```python
from build123d import *

# Parameters (mm, degrees)
SM_BASE_FLANGE_1_DEPTH            = 3
SM_EDGE_FLANGE_1_STRIP_W          = 13.4732
SM_EDGE_FLANGE_1_STRIP_H          = 3
SM_EDGE_FLANGE_1_STRIP_CUT_DEPTH  = 65.533094289
SM_EDGE_FLANGE_1_RELIEF_W         = 14.9732
SM_EDGE_FLANGE_1_RELIEF_H         = 1.5
SM_EDGE_FLANGE_1_RELIEF_CUT_DEPTH = 3
SM_EDGE_FLANGE_1_DEPTH            = 65.533094289
CHAMFER_1_SIZE                    = 5
CUT_EXTRUDE_1_DEPTH               = 10


# Sheet-metal steps are written as plain solids
with BuildPart() as part:
    # Sketch 1 → 基体-法兰1 (new body)
    with BuildSketch(Plane.XY):
        Polygon((75, -35), (75, -85.533094289), (95, -85.533094289), (95, 0), (0, 0), (0, -35), align=None)
    extrude(amount=-SM_BASE_FLANGE_1_DEPTH)

    # 边线-法兰1 strip (across the edge) → 边线-法兰1 strip cut (cut)
    with BuildSketch(Plane(origin=(95, -85.533094289, 0), x_dir=(-1, 0, 0), z_dir=(0, 1, 0))):
        with Locations((-3, -1.5)):
            Rectangle(SM_EDGE_FLANGE_1_STRIP_W, SM_EDGE_FLANGE_1_STRIP_H)
    extrude(amount=SM_EDGE_FLANGE_1_STRIP_CUT_DEPTH, mode=Mode.SUBTRACT)

    # 边线-法兰1 relief (on the sheet) → 边线-法兰1 relief cut (cut)
    with BuildSketch(Plane(origin=(91.2634, -85.533094289, 0), x_dir=(-1, 0, 0), z_dir=(0, 0, 1))):
        with Locations((-5.9866, -66.283094289)):
            Rectangle(SM_EDGE_FLANGE_1_RELIEF_W, SM_EDGE_FLANGE_1_RELIEF_H)
    extrude(amount=-SM_EDGE_FLANGE_1_RELIEF_CUT_DEPTH, mode=Mode.SUBTRACT)

    # 边线-法兰1 section (across the edge) → 边线-法兰1 (add)
    with BuildSketch(Plane(origin=(95, -85.533094289, 0), x_dir=(-1, 0, 0), z_dir=(0, 1, 0))):
        with BuildLine():
            Line((0, 0.7366), (0, 27))
            Line((0, 27), (3, 27))
            Line((3, 27), (3, 0.7366))
            ThreePointArc((3, 0.7366), (3.215745145, 0.215745145), (3.7366, 0))
            Line((3.7366, 0), (3.7366, -3))
            ThreePointArc((3.7366, -3), (1.094424801, -1.905575199), (0, 0.7366))
        make_face()
    extrude(amount=SM_EDGE_FLANGE_1_DEPTH)

    # 倒角1
    chamfer_1_edges = [part.edges().sort_by_distance(p)[0] for p in [
        (0, 0, -1.5),
        (95, 0, -1.5),
        (75, -85.533094289, -1.5),
        (0, -35, -1.5),
        (93.5, -85.533094289, 27),
        (93.5, -20, 27),
    ]]
    chamfer(chamfer_1_edges, length=CHAMFER_1_SIZE)

    # 草图10 → 切除-拉伸1 (cut)
    with BuildSketch(Plane.XY):
        with BuildLine():
            Line((11, -14), (19, -14))
            ThreePointArc((19, -14), (22.5, -17.5), (19, -21))
            Line((19, -21), (11, -21))
            ThreePointArc((11, -21), (7.5, -17.5), (11, -14))
        make_face()
        with BuildLine():
            Line((51, -14), (59, -14))
            ThreePointArc((59, -14), (62.5, -17.5), (59, -21))
            Line((59, -21), (51, -21))
            ThreePointArc((51, -21), (47.5, -17.5), (51, -14))
        make_face()
    extrude(amount=-CUT_EXTRUDE_1_DEPTH, mode=Mode.SUBTRACT)


solid = part.part
```
Check sheet for the modelled part. Datum: model origin and axes. Units: mm. A direction names the side the tool comes from. Give positions to 0.01 mm unless a question says otherwise; leave off trailing zeros. Order: outer loops, then holes, each group sorted by start corner. A loop starts at its lowest first (then second) coordinate and runs counter-clockwise, first axis right, second up. Notation, with made-up numbers: (2.5, -17) -> (15.5, -17) arc R17 cw to (15.5, 7) -> close; hole circle Ø4 at (89, -23.75). An arc over 180 degrees is marked (long way). Return JSON: item names as keys, results as strings.
1. Mould release check, pull along Y, two halves, no side actions. Record for faces 1 (the flat face through (55, -21, -1)), 2 (the cylindrical face through (93.88, -53.23, -1.93)), 3 (the flat face through (3, -2, -1)): +Y half, -Y half, draft (parallel to the pull), parting line (faces both ways), or undercut.
From the geometry:
{"face 1": "undercut", "face 2": "draft", "face 3": "+Y half"}
2. Cross-section at A-A, the plane x = 16. Record the cut outline in (y, z).
From the geometry:
{"outline": "(-35, -3) -> (-21, -3) -> (-21, 0) -> (-35, 0) -> close; (-14, -3) -> (0, -3) -> (0, 0) -> (-14, 0) -> close"}
3. Cross-section at C-C, the plane z = 11.5. Record the cut outline in (x, y), plus the area to 3 significant figures.
From the geometry:
{"outline": "(92, -85.53) -> (95, -85.53) -> (95, -20) -> (92, -20) -> close", "area": "197 mm^2"}
4. Set-up check for faces 4 (the flat face through (15, -21, -1)), 5 (the flat face through (94, -20, 10)), 6 (the flat face through (75, -57, -1)), 7 (the flat face through (92, -53, 14)), 8 (the flat face through (94, -22, 24)): record each of +Z, -Z, +X, -X, +Y, -Y from which the full face is reachable in a straight line by a thin tool's end or side.
From the geometry:
{"face 4": "+Z, -Z", "face 5": "+Z, -Z, +X", "face 6": "+Z, -Z, -X, -Y", "face 7": "+Z, -X, +Y, -Y", "face 8": "+Z, +X, -X, +Y"}
5. Go/stop test with flat-tipped pins: P1, Ø3.5, axis at x = 56, z = -1, coming from the -Y side; P2, Ø1.6, axis at x = 91.5, z = 4, coming from the +Y side; P3, Ø2, axis at y = -9, z = 2, coming from the +X side; P4, Ø5, axis at y = -56, z = 20.5, coming from the -X side. Record where each tip stops, or that it passes through.
From the geometry:
{"P1": "y = -35", "P2": "y = -20", "P3": "through", "P4": "x = 92"}
6. Cross-section at D-D, the plane y = -10. Record the cut outline in (x, z), plus the area to 3 significant figures.
From the geometry:
{"outline": "(0, -3) -> (95, -3) -> (95, 0) -> (0, 0) -> close", "area": "285 mm^2"}
7. Cross-section at B-B, the plane y = -50. Record the cut outline in (x, z), plus the area to 3 significant figures.
From the geometry:
{"outline": "(75, -3) -> (91.26, -3) arc R3.74 ccw to (95, 0.74) -> (95, 27) -> (92, 27) -> (92, 0.74) arc R0.74 cw to (91.26, 0) -> (75, 0) -> close", "area": "138 mm^2"}
8. Material ranges on probe 1 along Z at (x, y) = (52.5, -11); probe 2 along X at (y, z) = (-43, 9.75); probe 3 along X at (y, z) = (-69.5, -0.25), recorded low to high. Write a range as [from, to].
From the geometry:
{"probe 1": "[-3, 0]", "probe 2": "[92, 95]", "probe 3": "[75, 94.87]"}
